Here's how the part is built. I have some questions about the finished solid (model axes, mm). Face numbers are marked on the shaded views. A direction names the side the tool comes from. Give positions to 0.01 mm unless a question says otherwise; leave off trailing zeros. Order: outer loops, then holes, each group sorted by start corner. A loop starts at its lowest first (then second) coordinate and runs counter-clockwise, first axis right, second up. Notation, with made-up numbers: (58.5, 75) - (66.5, 75) arc R20 cw to (66.5, 79) - close; hole circle Ø9 at (17.5, -24). An arc over 180 degrees is marked (long way). One line per question, with ' | ' between items.
Autodesk Inventor part; units mm, degrees
sketch "Skizze1" plane through (0, 0, 0) normal (0, 0, 1) x (1, 0, 0)
  line L0 (0, 0) -> (42.19, 0)
  line L1 (2.6, 0) -> (2.6, 10)
  line L2 (39.89, 0) -> (39.89, 10)
  line L3 (2.6, 10) -> (39.89, 10)
  line L4 (0, 0) -> (-0.1073, 1.8337) construction
  spline S0 degree 3 poles (0, 0) (-0.1073, 1.8337) (0.0261, 2.9533) (0.334, 3.6563) knots 1 1 1 1 1.405888 1.405888 1.405888 1.405888
  line L5 (42.19, 0) -> (42.2285, 1.1988) construction
  spline S1 degree 3 poles (42.19, 0) (42.2285, 1.1988) (42.1183, 2.1671) (41.8072, 2.9533) knots 1 1 1 1 1.467938 1.467938 1.467938 1.467938
  line L6 (2.6, 10) -> (0.334, 3.6563)
  line L7 (-0.1073, 1.8337) -> (0.0261, 2.9533) construction
  line L8 (0.0261, 2.9533) -> (0.334, 3.6563) construction
  line L9 (39.89, 10) -> (41.8072, 2.9533)
  line L10 (42.2285, 1.1988) -> (42.1183, 2.1671) construction
  line L11 (42.1183, 2.1671) -> (41.8072, 2.9533) construction
  point P0 (39.89, 5)
  point P1 (2.6, 5)
  dimension "d0" = 42.19
  dimension "d1" = 2.6
  dimension "d2" = 10
  dimension "d3" = 2.3
extrude "Extrusion1" add sketch "Skizze1" along normal blind 52.21
sketch "Skizze3" plane through (0, 0, 0) normal (0, -1, 0) x (1, 0, 0)
  line L0 (0, 0) -> (42.19, 0)
  line L1 (0, 52.21) -> (42.19, 52.21)
  line L2 (42.19, 0) -> (42.19, 52.21)
  line L3 (0, 0) -> (0, 52.21)
  point P0 (21.095, 26.105)
hole "Bohrung2" at (21.095, 0, 26.105) direction (0, 1, 0) diameter 6.6 depth 10 counterbore diameter 15 counterbore depth 6
sketch "Skizze4" plane through (2.6, 10, 0) normal (0, 1, 0) x (1, 0, 0)
  line L0 (3.3345, -3.2969) -> (34.5895, -3.2969)
  line L1 (34.5895, -3.2969) -> (34.5895, -15.1659)
  line L2 (34.5895, -15.1659) -> (3.3345, -15.1659)
  line L3 (3.3345, -15.1659) -> (3.3345, -3.2969)
  circle A0 centre (18.495, -26.105) radius 3.3
  line L4 (37.29, 0) -> (0, 0)
  line L5 (0, 0) -> (0, -52.21)
  line L6 (37.29, -52.21) -> (0, -52.21)
  line L7 (37.29, 0) -> (37.29, -52.21)
  line L8 (18.495, -26.105) -> (-9.8533, -26.105)
  line L9 (3.3345, -48.9131) -> (34.5895, -48.9131)
  line L10 (34.5895, -48.9131) -> (34.5895, -37.0441)
  line L11 (34.5895, -37.0441) -> (3.3345, -37.0441)
  line L12 (3.3345, -37.0441) -> (3.3345, -48.9131)
  point P0 (-2.6, 0)
extrude "Extrusion2" cut sketch "Skizze4" against normal through all contours L0 L1 L2 L3 | L12 L11 L10 L9
properties part number "tripodInlay"
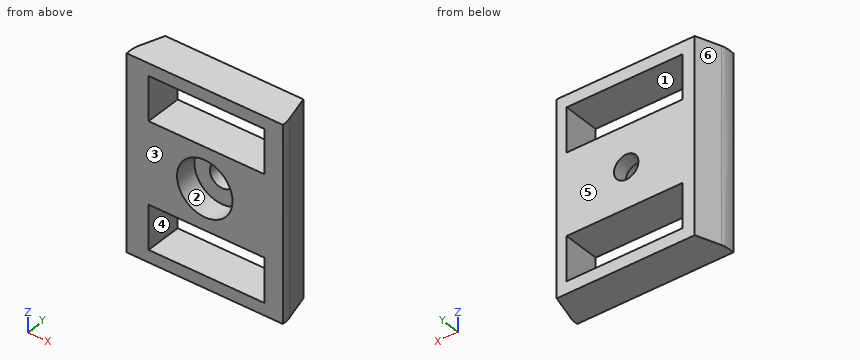
1) Please list where these lines run through material, in increasing order: L1, parallel to Z at x = 35, y = 7.25; L2, parallel to Z at x = 18, y = 0.75; L3, parallel to X at y = 5.75, z = 11.
Model answer:
L1: z = 0 to 3.3, 15.17 to 37.04, 48.91 to 52.21 | L2: z = 0 to 3.3, 15.17 to 19.27, 32.94 to 37.04, 48.91 to 52.21 | L3: x = 1.08 to 5.93, 37.19 to 41.05
2) I want a section at A-A (x = 11). List the corners of the cut face in (y, z) for me, plus the area to 3 significant figures.
Model answer:
outline: (0, 0) - (10, 0) - (10, 3.3) - (0, 3.3) - close; (0, 15.17) - (10, 15.17) - (10, 37.04) - (0, 37.04) - close; (0, 48.91) - (10, 48.91) - (10, 52.21) - (0, 52.21) - close | area: 285 mm2
3) On a 3-axis mill with a long thin cutter (end or side, diameter ignored), from which of +Z, -Z, +X, -X, +Y, -Y can I reach the whole of each face in a straight line? I mean the marked faces 1, 2 and 3. Say none if no direction works.
Model answer:
face 1: +Y, -Y | face 2: -Y | face 3: +Z, -Z, +X, -X, -Y
4) I want a section at C-C (x = 20.5). List the corners of the cut face in (y, z) for me, plus the area to 3 significant figures.
Model answer:
outline: (0, 0) - (10, 0) - (10, 3.3) - (0, 3.3) - close; (0, 15.17) - (10, 15.17) - (10, 22.86) - (6, 22.86) - (6, 18.63) - (0, 18.63) - close; (0, 33.58) - (6, 33.58) - (6, 29.35) - (10, 29.35) - (10, 37.04) - (0, 37.04) - close; (0, 48.91) - (10, 48.91) - (10, 52.21) - (0, 52.21) - close | area: 169 mm2
5) I want a section at B-B (y = 9). List the corners of the cut face in (x, z) for me (1 decimal), plus the area to 3 significant figures.
Model answer:
outline: (2.2, 0) - (40.2, 0) - (40.2, 52.2) - (2.2, 52.2) - close; hole (5.9, 3.3) - (37.2, 3.3) - (37.2, 15.2) - (5.9, 15.2) - close; hole (5.9, 37) - (37.2, 37) - (37.2, 48.9) - (5.9, 48.9) - close; hole circle Ø6.6 at (21.1, 26.1) | area: 1,200 mm2
6) Thinking about a two-plate mould opening in X: for the marked faces 4, 5 and 6, which applies, +X half, -X half, draft (parallel to the pull), parting line (faces both ways), or undercut?
Model answer:
face 4: undercut | face 5: draft | face 6: -X half
7) I'm going to push flat-ended pins straight in: P1, Ø10.5, axis at x = 21.095, z = 26.105, coming from the -Y side; P2, Ø2, axis at y = 7.5, z = 12, coming from the -X side; P3, Ø5, axis at y = 5, z = 45, coming from the +X side. Where does each tip first touch, or does it pass through?
Model answer:
P1: stops at y = 6 | P2: stops at x = 1.35 | P3: stops at x = 41.96
8) I want a section at D-D (y = 2). State how many separate pieces and enclosed holes the cut face has, plus the area to 3 significant figures.
Model answer:
separate pieces: 1 | enclosed holes: 3 | area: 1,280 mm2
